Check sheet for the modelled part. Datum: model origin and axes. Units: mm. A direction names the side the tool comes from. Round coordinates to 2 decimals unless told otherwise and drop trailing zeros. Order: outer loops, then holes, each group sorted by start corner. A loop starts at its lowest first (then second) coordinate and runs counter-clockwise, first axis right, second up.
Q1. Cross-section at A-A on x = 17.5. Record the cut outline in (y, z).
Q2. Cross-section at C-C on x = -35.9. Record the cut outline in (y, z), then the cut area to 3 significant figures.
Q3. Scan lines: probe 1 along Z at (x, y) = (-35.9, 2); probe 2 along Y at (x, z) = (-41.65, -27.05) (3 decimals); probe 3 along Z at (x, y) = (-35.9, 3.85). Record each from-to range of solid material in increasing order.
Q4. Cross-section at B-B on y = 47. Record the cut outline in (x, z).
Q5. Depth check by flat-ended pin: P1, Ø5, axis at x = -35.5, z = -22, coming from the +Y side; P2, Ø8, axis at y = 17.375, z = -18.5, coming from the +X side. Enter the tip coordinate at first touch or a pass-through.
Q6. Mould release check, pull along Z, two halves, no side actions. Record for faces 6 (the flat face through (-31.15, 18, 29)), 7 (the cylindrical face through (35.25, 4.73, -21.87)), 8 (the flat face through (9, 27, -46.15)): +Z half, -Z half, draft (parallel to the pull), parting line (faces both ways), or undercut.
Q7. Cross-section at D-D on z = 19.5. Record the cut outline in (x, y), then the cut area to 3 significant figures.
Q8. Set-up check for faces 1 (the cylindrical face through (-42.529, 33.546, -41.219)), 2 (the flat face through (-44.05, 25, -9)), 3 (the flat face through (9, 27, 27.95)), 4 (the cylindrical face through (62.529, 8.675, -7.014)), 5 (the flat face through (8.45, 18, 29)): record each of +Z, -Z, +X, -X, +Y, -Y from which the full face is reachable in a straight line by a thin tool's end or side.
from build123d import *

# Parameters (mm, degrees)
SKETCH1_W                 = 78.1
SKETCH1_H                 = 55.9
BOSS_EXTRUDE1_DEPTH       = 3
SKETCH2_R                 = 1.25
CUT_EXTRUDE1_DEPTH        = 68
SKETCH4_W                 = 82.1
SKETCH4_H                 = 59.9
SKETCH4_W_2               = 78.1
SKETCH4_H_2               = 55.9
BOSS_EXTRUDE3_DEPTH       = 3
SKETCH6_R                 = 3
SKETCH6_R_2               = 1.25
BOSS_EXTRUDE4_DEPTH       = 3.5
SKETCH7_W                 = 82.1
SKETCH7_H                 = 16.2
BOSS_EXTRUDE5_DEPTH       = 3
SKETCH8_W                 = 82.1
SKETCH8_H                 = 50.5
BOSS_EXTRUDE6_DEPTH       = 3
BOSS_EXTRUDE7_DEPTH       = 20
SKETCH12_W                = 79.1
SKETCH12_H                = 50.5
BOSS_EXTRUDE8_DEPTH       = 3
SKETCH17_W                = 105.1
SKETCH17_H                = 50.5
BOSS_EXTRUDE13_DEPTH      = 1
BOSS_EXTRUDE13_DEPTH_BACK = 2
SKETCH18_W                = 11.5
SKETCH18_H                = 7.7
SKETCH18_W_2              = 39.6
SKETCH18_H_2              = 9
CUT_EXTRUDE4_DEPTH        = 9
SKETCH19_W                = 80.1
SKETCH19_H                = 50.5
BOSS_EXTRUDE14_DEPTH      = 3
SKETCH20_R                = 19
SKETCH20_R_2              = 1.5
CUT_EXTRUDE5_DEPTH        = 3
SKETCH22_R                = 2.5
CUT_EXTRUDE6_DEPTH        = 3


with BuildPart() as part:
    # Sketch1 → Boss-Extrude1 (new body)
    with BuildSketch(Plane(origin=(0, 0, 0), x_dir=(1, 0, 0), z_dir=(0, 1, 0))):
        Rectangle(SKETCH1_W, SKETCH1_H)
    extrude(amount=BOSS_EXTRUDE1_DEPTH)

    # Sketch2 → Cut-Extrude1 (cut)
    with BuildSketch(Plane(origin=(0, 3, 0), x_dir=(1, 0, 0), z_dir=(0, 1, 0))):
        with Locations((-35.9, 20.9)):
            Circle(SKETCH2_R)
        with Locations((-35.9, -24.8)):
            Circle(SKETCH2_R)
        with Locations((35.9, -24.8)):
            Circle(SKETCH2_R)
        with Locations((35.9, 24.8)):
            Circle(SKETCH2_R)
    extrude(amount=-CUT_EXTRUDE1_DEPTH, mode=Mode.SUBTRACT)

    # Sketch4 → Boss-Extrude3 (add)
    with BuildSketch(Plane(origin=(0, 0, 0), x_dir=(-1, 0, 0), z_dir=(0, -1, 0))):
        Rectangle(SKETCH4_W, SKETCH4_H)
        Rectangle(SKETCH4_W_2, SKETCH4_H_2, mode=Mode.SUBTRACT)
    extrude(amount=-BOSS_EXTRUDE3_DEPTH)

    # Sketch6 → Boss-Extrude4 (add)
    with BuildSketch(Plane(origin=(0, 3, 0), x_dir=(1, 0, 0), z_dir=(0, 1, 0))):
        with Locations((-35.9, 20.9)):
            Circle(SKETCH6_R)
        with Locations((-35.9, 20.9)):
            Circle(SKETCH6_R_2, mode=Mode.SUBTRACT)
        with Locations((35.9, 24.8)):
            Circle(SKETCH6_R)
        with Locations((35.9, 24.8)):
            Circle(SKETCH6_R_2, mode=Mode.SUBTRACT)
        with Locations((35.9, -24.8)):
            Circle(SKETCH6_R)
        with Locations((35.9, -24.8)):
            Circle(SKETCH6_R_2, mode=Mode.SUBTRACT)
        with Locations((-35.9, -24.8)):
            Circle(SKETCH6_R)
        with Locations((-35.9, -24.8)):
            Circle(SKETCH6_R_2, mode=Mode.SUBTRACT)
    extrude(amount=BOSS_EXTRUDE4_DEPTH)

    # Sketch7 → Boss-Extrude5 (add)
    with BuildSketch(Plane(origin=(0, 0, 0), x_dir=(-1, 0, 0), z_dir=(0, -1, 0))):
        with Locations((0, 38.05)):
            Rectangle(SKETCH7_W, SKETCH7_H)
    extrude(amount=-BOSS_EXTRUDE5_DEPTH)

    # Sketch8 → Boss-Extrude6 (add)
    with BuildSketch(Plane(origin=(0, 0, -46.15), x_dir=(-1, 0, 0), z_dir=(0, 0, -1))):
        with Locations((0, 25.25)):
            Rectangle(SKETCH8_W, SKETCH8_H)
    extrude(amount=BOSS_EXTRUDE6_DEPTH)

    # Sketch10 → Boss-Extrude7 (add)
    with BuildSketch(Plane(origin=(41.05, 0, 0), x_dir=(0, 0, -1), z_dir=(1, 0, 0))):
        Polygon((49.15, 50.5), (46.15, 50.5), (46.15, 3), (-29.95, 3), (-29.95, 0), (49.15, 0), align=None)
    extrude(amount=BOSS_EXTRUDE7_DEPTH)

    # Sketch12 → Boss-Extrude8 (add)
    with BuildSketch(Plane.ZY.offset(41.05)):
        with Locations((-9.6, 25.25)):
            Rectangle(SKETCH12_W, SKETCH12_H)
    extrude(amount=BOSS_EXTRUDE8_DEPTH)

    # Sketch17 → Boss-Extrude13 (add, two sides)
    with BuildSketch(Plane.XY.offset(29.95)) as boss_extrude13_sk:
        with Locations((8.5, 25.25)):
            Rectangle(SKETCH17_W, SKETCH17_H)
    extrude(amount=BOSS_EXTRUDE13_DEPTH)
    extrude(boss_extrude13_sk.sketch, amount=-BOSS_EXTRUDE13_DEPTH_BACK)

    # Sketch18 → Cut-Extrude4 (cut)
    with BuildSketch(Plane(origin=(0, 0, 27.95), x_dir=(-1, 0, 0), z_dir=(0, 0, -1))):
        with Locations((-21.6, 9.95)):
            Rectangle(SKETCH18_W, SKETCH18_H)
        with Locations((11.35, 17.6)):
            Rectangle(SKETCH18_W_2, SKETCH18_H_2)
    extrude(amount=-CUT_EXTRUDE4_DEPTH, mode=Mode.SUBTRACT)

    # Sketch19 → Boss-Extrude14 (add)
    with BuildSketch(Plane(origin=(61.05, 0, 0), x_dir=(0, 0, -1), z_dir=(1, 0, 0))):
        with Locations((9.1, 25.25)):
            Rectangle(SKETCH19_W, SKETCH19_H)
    extrude(amount=BOSS_EXTRUDE14_DEPTH)

    # Sketch20 → Cut-Extrude5 (cut)
    with BuildSketch(Plane.ZY.offset(-61.05)):
        with Locations((-24.15, 25)):
            Circle(SKETCH20_R)
        with Locations((-8.4, 40.75)):
            Circle(SKETCH20_R_2)
        with Locations((-39.9, 40.75)):
            Circle(SKETCH20_R_2)
        with Locations((-8.4, 9.25)):
            Circle(SKETCH20_R_2)
        with Locations((-39.9, 9.25)):
            Circle(SKETCH20_R_2)
    extrude(amount=-CUT_EXTRUDE5_DEPTH, mode=Mode.SUBTRACT)

    # Sketch22 → Cut-Extrude6 (cut)
    with BuildSketch(Plane(origin=(-41.05, 0, 0), x_dir=(0, 0, -1), z_dir=(1, 0, 0))):
        with Locations((14.225, 12.6875)):
            Circle(SKETCH22_R)
        with Locations((14.225, 22.0625)):
            Circle(SKETCH22_R)
        with Locations((18.5, 17.375)):
            Circle(SKETCH22_R)
        with Locations((22.775, 22.0625)):
            Circle(SKETCH22_R)
        with Locations((22.775, 12.6875)):
            Circle(SKETCH22_R)
        with Locations((14.225, 31.4375)):
            Circle(SKETCH22_R)
        with Locations((18.5, 26.75)):
            Circle(SKETCH22_R)
        with Locations((22.775, 31.4375)):
            Circle(SKETCH22_R)
        with Locations((18.5, 36.125)):
            Circle(SKETCH22_R)
        with Locations((14.225, 40.8125)):
            Circle(SKETCH22_R)
        with Locations((22.775, 40.8125)):
            Circle(SKETCH22_R)
        with Locations((27.05, 36.125)):
            Circle(SKETCH22_R)
        with Locations((31.325, 40.8125)):
            Circle(SKETCH22_R)
        with Locations((39.875, 40.8125)):
            Circle(SKETCH22_R)
        with Locations((35.6, 36.125)):
            Circle(SKETCH22_R)
        with Locations((39.875, 31.4375)):
            Circle(SKETCH22_R)
        with Locations((31.325, 31.4375)):
            Circle(SKETCH22_R)
        with Locations((27.05, 26.75)):
            Circle(SKETCH22_R)
        with Locations((31.325, 22.0625)):
            Circle(SKETCH22_R)
        with Locations((39.875, 22.0625)):
            Circle(SKETCH22_R)
        with Locations((35.6, 26.75)):
            Circle(SKETCH22_R)
        with Locations((27.05, 17.375)):
            Circle(SKETCH22_R)
        with Locations((31.325, 12.6875)):
            Circle(SKETCH22_R)
        with Locations((39.875, 12.6875)):
            Circle(SKETCH22_R)
        with Locations((35.6, 17.375)):
            Circle(SKETCH22_R)
        with Locations((18.5, 8)):
            Circle(SKETCH22_R)
        with Locations((27.05, 8)):
            Circle(SKETCH22_R)
        with Locations((35.6, 8)):
            Circle(SKETCH22_R)
    extrude(amount=-CUT_EXTRUDE6_DEPTH, mode=Mode.SUBTRACT)


solid = part.part
Results found:
1. outline: (0, -49.15) - (50.5, -49.15) - (50.5, -46.15) - (3, -46.15) - (3, 27.95) - (6.1, 27.95) - (6.1, 30.95) - (0, 30.95) - close; (13.8, 27.95) - (50.5, 27.95) - (50.5, 30.95) - (13.8, 30.95) - close
2. outline: (0, -49.15) - (50.5, -49.15) - (50.5, -46.15) - (3, -46.15) - (3, -23.9) - (6.5, -23.9) - (6.5, -22.15) - (0, -22.15) - close; (0, -19.65) - (6.5, -19.65) - (6.5, -17.9) - (3, -17.9) - (3, 21.8) - (6.5, 21.8) - (6.5, 23.55) - (0, 23.55) - close; (0, 26.05) - (6.5, 26.05) - (6.5, 27.8) - (3, 27.8) - (3, 27.95) - (50.5, 27.95) - (50.5, 30.95) - (0, 30.95) - close
2. area: 535 mm2
3. probe 1: z = -49.15 to -22.15, -19.65 to 23.55, 26.05 to 30.95
3. probe 2: y = 0 to 5.5, 10.5 to 14.875, 19.875 to 24.25, 29.25 to 33.625, 38.625 to 50.5
3. probe 3: z = -49.15 to -46.15, -23.9 to -22.15, -19.65 to -17.9, 21.8 to 23.55, 26.05 to 27.8, 27.95 to 30.95
4. outline: (-44.05, -49.15) - (64.05, -49.15) - (64.05, 30.95) - (-44.05, 30.95) - close; hole (-41.05, -46.15) - (61.05, -46.15) - (61.05, 27.95) - (-41.05, 27.95) - close
5. P1: stops at y = 6.5
5. P2: stops at x = -41.05
6. face 6: draft
6. face 7: undercut
6. face 8: undercut
7. outline: (-44.05, 0) - (64.05, 0) - (64.05, 50.5) - (61.05, 50.5) - (61.05, 3) - (-41.05, 3) - (-41.05, 50.5) - (-44.05, 50.5) - close
7. area: 609 mm2
8. face 1: -X
8. face 2: +Z, -Z, -X, +Y, -Y
8. face 3: +Y
8. face 4: +X
8. face 5: +Z
